Drawing for the job (mm, zero at the part's lowest x, y, z). A direction names the side the tool comes from. Give positions to 0.01 mm unless a question says otherwise; leave off trailing zeros. Write each loop counter-clockwise with the first axis right and the second up, starting at its lowest first coordinate (ties: lowest second). Pieces come first, ordered by that corner, then holes. Notation, with made-up numbers: M 84.5,-27.5 L 124.5,-27.5 A34 cw 124.5,2.5 Z; hole C 53.25,32 d9. An arc over 180 degrees is marked long. Use a Markdown table: item, result. Add a question column.
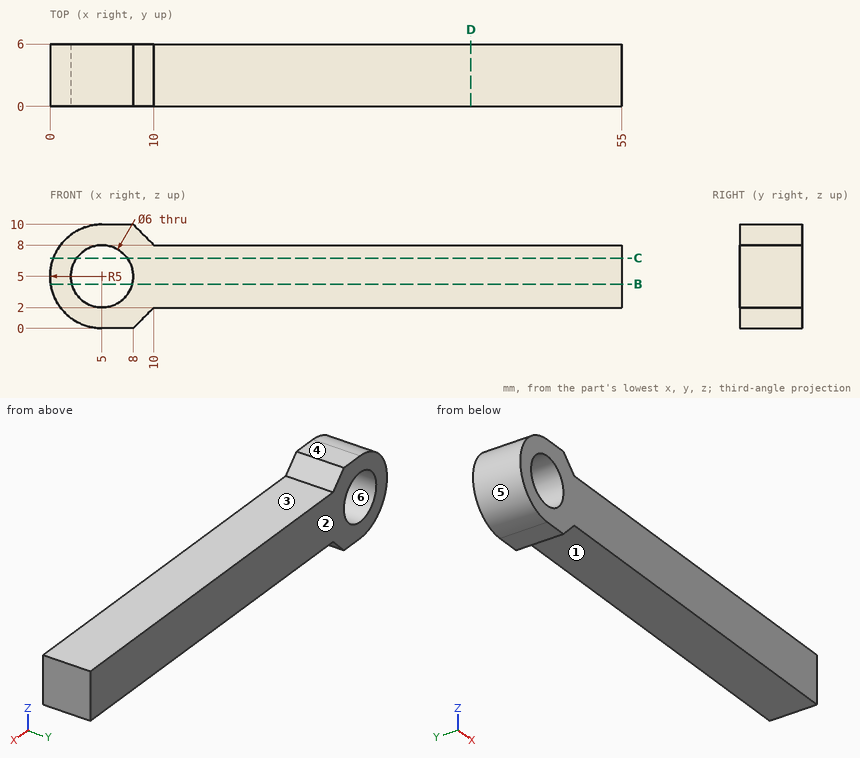
1. Mould opens along Z. For the marked faces 4, 5 and 6 say: released by +Z, released by -Z, zero draft, split by the parting line, or undercut.
2. Cut at D-D (x = 40.5). Write the cut outline in (y, z).
3. Cut at B-B (z = 4.25). Write the cut outline in (x, y), then the cut area to 3 significant figures.
4. Drill centre lines: probe 1 along X at (y, z) = (2.15, 5); probe 2 along Z at (x, y) = (5, 2.45); probe 3 along Z at (x, y) = (32, 2). Where is each one in solid material? Low to high. Write a range as [from, to].
5. Cut at C-C (z = 6.75). Write the cut outline in (x, y), then the cut area to 3 significant figures.
6. Tool access for the marked faces 1, 2 and 3: list every direction of +Z, -Z, +X, -X, +Y, -Y with a clear straight run to the whole face (end or side of a thin tool).
7. Flat gauge pins, fed straight in: pin 1 (1.8 mm diameter, centred on x = 32.5, y = 3, fed in from +Z); pin 2 (3 mm diameter, centred on x = 13, z = 1, fed in from -Y); pin 3 (3 mm diameter, centred on x = 33.5, y = 3.5, fed in from -Z). Where does each tip first touch, or does it go through?
A:
| question | item | result |
|---|---|---|
| 1 | face 4 | released by +Z |
| 1 | face 5 | split by the parting line |
| 1 | face 6 | undercut |
| 2 | outline | M 0,2 L 6,2 L 6,8 L 0,8 Z |
| 3 | outline | M 0.06,0 L 2.1,0 L 2.1,6 L 0.06,6 Z; M 7.9,0 L 55,0 L 55,6 L 7.9,6 Z |
| 3 | area | 295 mm² |
| 4 | probe 1 | x = [0, 2], [8, 55] |
| 4 | probe 2 | z = [0, 2], [8, 10] |
| 4 | probe 3 | z = [2, 8] |
| 5 | outline | M 0.32,0 L 2.56,0 L 2.56,6 L 0.32,6 Z; M 7.44,0 L 55,0 L 55,6 L 7.44,6 Z |
| 5 | area | 299 mm² |
| 6 | face 1 | -Z, +X, +Y, -Y |
| 6 | face 2 | +Z, -Z, +X, -X, +Y |
| 6 | face 3 | +Z, +X, +Y, -Y |
| 7 | pin 1 | stops at z = 8 |
| 7 | pin 2 | stops at y = 0 |
| 7 | pin 3 | stops at z = 2 |
